```python
from build123d import *

# Parameters (mm, degrees)
SKETCH001_W  = 95.18
SKETCH001_H  = 25.4
PAD_DEPTH    = 2
SKETCH_R     = 1.26
PAD001_DEPTH = 3


with BuildPart() as part:
    # Sketch001 → Pad (new body)
    with BuildSketch(Plane.XY):
        Rectangle(SKETCH001_W, SKETCH001_H)
    extrude(amount=-PAD_DEPTH)

    # Sketch → Pad001 (join)
    with BuildSketch(Plane.XY):
        with Locations((-45.05, 8.89)):
            Circle(SKETCH_R)
        with Locations((0.67, 8.89)):
            Circle(SKETCH_R)
        with Locations((-45.05, -8.89)):
            Circle(SKETCH_R)
        with Locations((0.67, -8.89)):
            Circle(SKETCH_R)
        with Locations((27.4, 10.16)):
            Circle(SKETCH_R)
        with Locations((27.4, -10.16)):
            Circle(SKETCH_R)
        with Locations((45.18, 10.16)):
            Circle(SKETCH_R)
        with Locations((45.18, -10.16)):
            Circle(SKETCH_R)
        with Locations((7.75, 10.16)):
            Circle(SKETCH_R)
        with Locations((20.45, 10.16)):
            Circle(SKETCH_R)
        with Locations((7.75, -10.16)):
            Circle(SKETCH_R)
        with Locations((20.45, -10.16)):
            Circle(SKETCH_R)
    extrude(amount=PAD001_DEPTH)


solid = part.part
```
Here's how the part is built. I have some questions about the finished solid (model axes, mm). A direction names the side the tool comes from. Coordinates: 2 decimals unless noted, no trailing zeros. Order: outer loops, then holes, each group sorted by start corner. A loop starts at its lowest first (then second) coordinate and runs counter-clockwise, first axis right, second up. Notation, with made-up numbers: (23.25, -30.5) - (58.25, -30.5) arc R27 cw to (58.25, 0.5) - close; hole circle Ø11 at (16, 40.5). An arc over 180 degrees is marked (long way). One line per question, with ' | ' between items. Start each with the question number.
1. If we section it at D-D (x = -12.5): Write out the boundary of the cut face in (y, z), and give its area (3 significant figures).
2. If we section it at B-B (x = -45.05): Write out the boundary of the cut face in (y, z), and give its area (3 significant figures).
3. If we section it at C-C (y = -4.75): Write out the boundary of the cut face in (x, z), and give its area (3 significant figures).
4. Please list where these lines run through material, in increasing order: line 1 along X through (y, z) = (-11.25, 2.05); line 2 along Z through (x, y) = (-18, 1.5); line 3 along Y through (x, z) = (0.5, 2.3). Write a range as [from, to].
5. If we section it at A-A (z = 1.75): Give the number of separate pieces and of enclosed holes in the cut face, and give its area (3 significant figures).
6. I'm going to push flat-ended pins straight in: pin 1 Ø8 at (x, y) = (-6, 2.5) entering from +Z; pin 2 Ø3 at (x, z) = (-5.5, 2) entering from +Y. Where does each tip first touch, or does it pass through?
7. If we mould it in two halves opening along X, with no side actions, what happens to faces 1 (the cylindrical face through (26.47, 11.01, 1.48)), 2 (the flat face through (8, -10, 3)), 3 (the cylindrical face through (46.38, 10.54, 1.48))? For each: released by +X, released by -X, zero draft, split by the parting line, or undercut.
8. Which directions (+Z, -Z, +X, -X, +Y, -Y) give clear straight access to the entire face, cutting with the end or side of a thin tool? Please do faces 4 (the flat face through (1, 9, 3)), 5 (the cylindrical face through (46.344, -10.643, 1.479)).
Model answer:
1) outline: (-12.7, -2) - (12.7, -2) - (12.7, 0) - (-12.7, 0) - close | area: 50.8 mm²
2) outline: (-12.7, -2) - (12.7, -2) - (12.7, 0) - (10.15, 0) - (10.15, 3) - (7.63, 3) - (7.63, 0) - (-7.63, 0) - (-7.63, 3) - (-10.15, 3) - (-10.15, 0) - (-12.7, 0) - close | area: 65.9 mm²
3) outline: (-47.59, -2) - (47.59, -2) - (47.59, 0) - (-47.59, 0) - close | area: 190 mm²
4) line 1: x = [7.12, 8.38], [19.82, 21.08], [26.77, 28.03], [44.55, 45.81] | line 2: z = [-2, 0] | line 3: y = [-10.14, -7.64], [7.64, 10.14]
5) separate pieces: 12 | enclosed holes: 0 | area: 59.9 mm²
6) pin 1: stops at z = 0 | pin 2: passes through
7) face 1: undercut | face 2: zero draft | face 3: undercut
8) face 4: +Z, +X, -X, +Y, -Y | face 5: +Z
